from build123d import *

# Parameters (mm, degrees)
SKETCH1_R       = 21
SIDE_1_DEPTH    = 2
SKETCH2_R       = 15
PULLEY_DEPTH    = 9
SKETCH3_R       = 21
SIDE_2_DEPTH    = 2
SKETCH4_R       = 4.8125
SHAFTHOLE_DEPTH = 13
SKETCH5_W       = 3
SKETCH5_H       = 4
KEYWAY_DEPTH    = 13
SKETCH6_R       = 1.25
CABLEHOLE_DEPTH = 2


with BuildPart() as part:
    # Sketch1 → Side 1 (new body)
    with BuildSketch(Plane.XY):
        Circle(SKETCH1_R)
    extrude(amount=SIDE_1_DEPTH)

    # Sketch2 → Pulley (add)
    with BuildSketch(Plane(origin=(0, 0, 0), x_dir=(-1, 0, 0), z_dir=(0, 0, -1))):
        Circle(SKETCH2_R)
    extrude(amount=PULLEY_DEPTH)

    # Sketch3 → Side 2 (add)
    with BuildSketch(Plane(origin=(0, 0, -9), x_dir=(-1, 0, 0), z_dir=(0, 0, -1))):
        Circle(SKETCH3_R)
    extrude(amount=SIDE_2_DEPTH)

    # Sketch4 → ShaftHole (cut)
    with BuildSketch(Plane(origin=(0, 0, -11), x_dir=(-1, 0, 0), z_dir=(0, 0, -1))):
        Circle(SKETCH4_R)
    extrude(amount=-SHAFTHOLE_DEPTH, mode=Mode.SUBTRACT)

    # Sketch5 → KeyWay (cut)
    with BuildSketch(Plane(origin=(0, 0, -11), x_dir=(-1, 0, 0), z_dir=(0, 0, -1))):
        with Locations((0, 4.8125)):
            Rectangle(SKETCH5_W, SKETCH5_H)
    extrude(amount=-KEYWAY_DEPTH, mode=Mode.SUBTRACT)

    # Sketch6 → CableHole (cut)
    with BuildSketch(Plane.XY.offset(2)):
        with Locations((17, 0)):
            Circle(SKETCH6_R)
        with Locations((16.420739047, 4.399923767)):
            Circle(SKETCH6_R)
    extrude(amount=-CABLEHOLE_DEPTH, mode=Mode.SUBTRACT)


solid = part.part
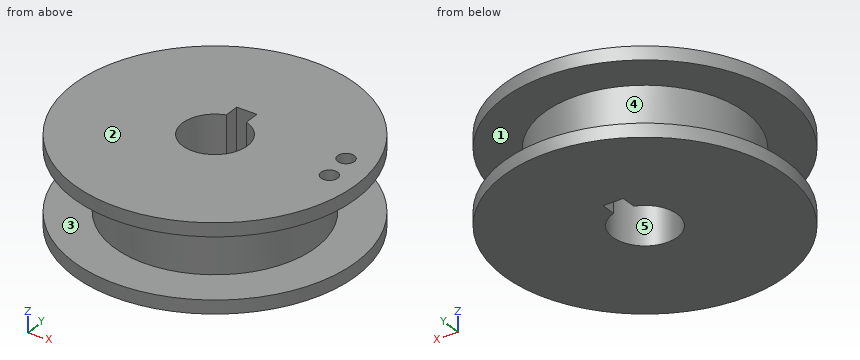
Source: CAD feature listing. Evaluate the final solid. Frame: model axes, mm. Face numbers are marked on the shaded views. A direction names the side the tool comes from. Give positions to 0.01 mm unless a question says otherwise; leave off trailing zeros. Loops run counter-clockwise (first coordinate to the right, second up) from the corner with the lowest first, then second, coordinate; pieces in that order, holes last. Notation, with made-up numbers: (-4.5, 41) -> (36.5, 41) arc R21 cw to (36.5, 68) -> close; hole circle Ø2 at (3.25, 3). An arc over 180 degrees is marked (long way). Use a Markdown table: item, result. Add a question column.
1) Section query D-D, the plane x = 17. Return the cut outline in (y, z), then the cut area to 3 significant figures.
2) Section query A-A, the plane x = 0. Return the cut outline in (y, z), then the cut area to 3 significant figures.
3) Reachability of the marked faces 1 and 2 from +Z, -Z, +X, -X, +Y, -Y: full face, straight path, thin tool, end or side. Return the list, or none.
4) First-contact query: pin 1 (3 mm diameter, centred on x = 1.5, z = 0.5, fed in from -Y); pin 2 (1.1 mm diameter, centred on y = 5.5, z = -2.5, fed in from -X); pin 3 (1.5 mm diameter, centred on y = 7.5, z = -7, fed in from +X); pin 4 (12 mm diameter, centred on x = -3, y = 1.5, fed in from +Z). Flat tips, straight axial feed; report the tip coordinate or a pass-through.
5) Section query C-C, the plane y = 17. Return the cut outline in (x, z).
6) Pull-direction query (X, two-part tool) for the marked faces 3, 4 and 5; classes: +X half, -X half, draft (parallel to the pull), parting line (faces both ways), or undercut.
7) Section query B-B, the plane z = -1.25. Return the cut outline in (x, y) (1 decimal).
8) Line query: line 1 along Z through (x, y) = (-17, -10); line 2 along X through (y, z) = (2.5, -3.5); line 3 along X through (y, z) = (13.5, -1.25). Output: solid intervals per line, ascending. Write a range as [from, to].
Numbers:
| question | item | result |
|---|---|---|
| 1 | outline | (-12.33, -11) -> (12.33, -11) -> (12.33, -9) -> (-12.33, -9) -> close; (-12.33, 0) -> (-1.25, 0) -> (-1.25, 2) -> (-12.33, 2) -> close; (1.25, 0) -> (3.29, 0) -> (3.29, 2) -> (1.25, 2) -> close; (5.51, 0) -> (12.33, 0) -> (12.33, 2) -> (5.51, 2) -> close |
| 1 | area | 89.2 mm2 |
| 2 | outline | (-21, -11) -> (-4.81, -11) -> (-4.81, 2) -> (-21, 2) -> (-21, 0) -> (-15, 0) -> (-15, -9) -> (-21, -9) -> close; (6.81, -11) -> (21, -11) -> (21, -9) -> (15, -9) -> (15, 0) -> (21, 0) -> (21, 2) -> (6.81, 2) -> close |
| 2 | area | 287 mm2 |
| 3 | face 1 | none |
| 3 | face 2 | +Z, +X, -X, +Y, -Y |
| 4 | pin 1 | stops at y = -21 |
| 4 | pin 2 | stops at x = -14.16 |
| 4 | pin 3 | stops at x = 13.4 |
| 4 | pin 4 | stops at z = 2 |
| 5 | outline | (-12.33, -11) -> (12.33, -11) -> (12.33, -9) -> (-12.33, -9) -> close; (-12.33, 0) -> (12.33, 0) -> (12.33, 2) -> (-12.33, 2) -> close |
| 6 | face 3 | draft |
| 6 | face 4 | parting line |
| 6 | face 5 | undercut |
| 7 | outline | circle Ø30 at (0, 0); hole (-1.5, 4.6) arc R4.8 ccw (long way) to (1.5, 4.6) -> (1.5, 6.8) -> (-1.5, 6.8) -> close |
| 8 | line 1 | z = [-11, -9], [0, 2] |
| 8 | line 2 | x = [-14.79, -4.11], [4.11, 14.79] |
| 8 | line 3 | x = [-6.54, 6.54] |
